CAD build for the part. Positions are in the model's coordinates, mm. A direction names the side the tool comes from. Give positions to 0.01 mm unless a question says otherwise; leave off trailing zeros. Loops run counter-clockwise (first coordinate to the right, second up) from the corner with the lowest first, then second, coordinate; pieces in that order, holes last. Notation, with made-up numbers: (63.5, 55) -> (112.5, 55) arc R23 cw to (112.5, 70) -> close; hole circle Ø3 at (58, 65). An arc over 180 degrees is marked (long way). Use one line per item in the form item = value.
```python
from build123d import *

# Parameters (mm, degrees)
F1_DEPTH = 12.7
F2_DEPTH = 2.54


with BuildPart() as f1:
    # F0 (on Front) → F1 (new body)
    with BuildSketch(Plane.XZ):
        with BuildLine():
            Line((63.5, 30.48), (-63.5, 30.48))
            ThreePointArc((-63.5, 30.48), (-93.98, 0), (-63.5, -30.48))
            Line((-63.5, -30.48), (63.5, -30.48))
            ThreePointArc((63.5, -30.48), (93.98, 0), (63.5, 30.48))
        make_face()
        with BuildLine():
            Line((63.5, -25.4), (-63.5, -25.4))
            ThreePointArc((-63.5, -25.4), (-88.9, 0), (-63.5, 25.4))
            Line((-63.5, 25.4), (63.5, 25.4))
            ThreePointArc((63.5, 25.4), (88.9, 0), (63.5, -25.4))
        make_face(mode=Mode.SUBTRACT)
    extrude(amount=F1_DEPTH)

    # F0 (on Front) → F2 (join)
    with BuildSketch(Plane.XZ):
        with BuildLine():
            Line((63.5, 30.48), (-63.5, 30.48))
            ThreePointArc((-63.5, 30.48), (-93.98, 0), (-63.5, -30.48))
            Line((-63.5, -30.48), (63.5, -30.48))
            ThreePointArc((63.5, -30.48), (93.98, 0), (63.5, 30.48))
        make_face()
        with BuildLine():
            Line((63.5, -25.4), (-63.5, -25.4))
            ThreePointArc((-63.5, -25.4), (-88.9, 0), (-63.5, 25.4))
            Line((-63.5, 25.4), (63.5, 25.4))
            ThreePointArc((63.5, 25.4), (88.9, 0), (63.5, -25.4))
        make_face(mode=Mode.SUBTRACT)
        with BuildLine():
            ThreePointArc((-63.5, 25.4), (-88.9, 0), (-63.5, -25.4))
            Line((-63.5, -25.4), (63.5, -25.4))
            ThreePointArc((63.5, -25.4), (88.9, 0), (63.5, 25.4))
            Line((63.5, 25.4), (-63.5, 25.4))
        make_face()
    extrude(amount=-F2_DEPTH)


solid = f1.part
```
1. Drill centre lines: line 1 (Z direction, x = 16.5, y = -6.75); line 2 (Y direction, x = 7, z = 0.5); line 3 (X direction, y = -8, z = 9.5). Where is each one in solid material? Low to high.
Result sheet:
line_1 = -30.48 to -25.4, 25.4 to 30.48
line_2 = 0 to 2.54
line_3 = -92.46 to -87.06, 87.06 to 92.46
2. Drop flat-ended pins along their axis: P1, Ø10, axis at x = -61.5, z = 13.5, coming from the -Y side; P2, Ø6, axis at x = 73, y = -4.5, coming from the +Z side. Give the stop position or say it passes through.
Result sheet:
P1 = 0
P2 = 29.78
3. Cut at B-B, the plane y = -3. Write the cut outline in (x, z).
Result sheet:
outline = (-63.5, -30.48) -> (63.5, -30.48) arc R30.48 ccw to (63.5, 30.48) -> (-63.5, 30.48) arc R30.48 ccw to start; hole (-63.5, -25.4) -> (63.5, -25.4) arc R25.4 ccw to (63.5, 25.4) -> (-63.5, 25.4) arc R25.4 ccw to start
4. Cut at A-A, the plane z = 0. Write the cut outline in (x, y).
Result sheet:
outline = (-93.98, -12.7) -> (-88.9, -12.7) -> (-88.9, 0) -> (88.9, 0) -> (88.9, -12.7) -> (93.98, -12.7) -> (93.98, 2.54) -> (-93.98, 2.54) -> close
5. Cut at C-C, the plane x = 51.5. Write the cut outline in (y, z).
Result sheet:
outline = (-12.7, -30.48) -> (2.54, -30.48) -> (2.54, 30.48) -> (-12.7, 30.48) -> (-12.7, 25.4) -> (0, 25.4) -> (0, -25.4) -> (-12.7, -25.4) -> close
6. Tool access for faces 4 (the flat face through (-1, -6, 25.4)), 5 (the flat face through (-1, -5, -30.48)): list every direction of +Z, -Z, +X, -X, +Y, -Y with a clear straight run to the whole face (end or side of a thin tool).
Result sheet:
face_4 = -Y
face_5 = -Z, +X, -X, +Y, -Y
7. Mould opens along X. For faces 1 (the flat face through (-1, 2.54, 0)), 2 (the cylindrical face through (93.973, -5.187, -0.67)), 3 (the flat face through (-1, 0, 0)) say: pulls with the +X half, pulls with the -X half, needs draft (parallel to the pull), parting line crosses it, or undercut.
Result sheet:
face_1 = needs draft
face_2 = pulls with the +X half
face_3 = undercut
